from build123d import *

# Parameters (mm, degrees)
F0_W     = 169.7224378586
F0_H     = 29.1480664164
F1_DEPTH = 5
F2_R     = 5
F3_DEPTH = 5.001
F6_R     = 5
F7_DEPTH = 5


# Not quite as in the source:
# - a feature of the source that left no trace in its solid (it failed there, or was rolled back) is left out


with BuildPart() as f1:
    # F0 (on Top) → F1 (new body)
    with BuildSketch(Plane.XY):
        with Locations((-209.8612189293, 14.5740332082)):
            Rectangle(F0_W, F0_H)
        Polygon((125, -249.6209740639), (125, -125), (-125, -125), (-125, 0), (-294.7224378586, 0), (-294.7224378586, -249.6209740639), align=None)
        Polygon((124.7859969735, -298.5799014568), (125, -249.6209740639), (-294.7224378586, -249.6209740639), (-294.7224378586, -298.5799014568), align=None)
    extrude(amount=F1_DEPTH)

    # F2 (on face) → F3 (cut, through all)
    with BuildSketch(Plane.XY.offset(5)):
        with Locations((-228.7230412454, -24.2026941362)):
            Circle(F2_R)
        with Locations((-219.7715429866, -67.8267564705)):
            Circle(F2_R)
        with Locations((-202.5809461153, -108.9080358424)):
            Circle(F2_R)
        with Locations((-177.7957154285, -145.9064206102)):
            Circle(F2_R)
        with Locations((-146.3450338267, -177.4348643144)):
            Circle(F2_R)
        with Locations((-109.4079678244, -202.3113851876)):
            Circle(F2_R)
        with Locations((-68.3692650785, -219.6033779172)):
            Circle(F2_R)
        with Locations((-24.7674410595, -228.6625764382)):
            Circle(F2_R)
        with Locations((19.7628989378, -229.1493570263)):
            Circle(F2_R)
        with Locations((63.5523401318, -221.0454705796)):
            Circle(F2_R)
    extrude(amount=-F3_DEPTH, mode=Mode.SUBTRACT)


with BuildPart() as f7:
    # F6 (on face) → F7 (new body)
    with BuildSketch(Plane.XY.offset(5)):
        with BuildLine():
            ThreePointArc((-44.6295934942, -213.8640500528), (-51.5484234193, -191.3776944906), (-69.9114028179, -176.6703024168))
            ThreePointArc((-69.9114028179, -176.6703024168), (-121.8233411216, -199.1458593545), (-99.3477842144, -251.0577976715))
            ThreePointArc((-99.3477842144, -251.0577976715), (-62.1432379515, -246.945220141), (-44.6295934942, -213.8640500528))
        make_face()
        with Locations((-109.4079678244, -202.3113851876)):
            Circle(F6_R, mode=Mode.SUBTRACT)
        with Locations((-68.3692650785, -219.6033779172)):
            Circle(F6_R, mode=Mode.SUBTRACT)
        with BuildLine():
            ThreePointArc((-139.8690317235, -128.5949220021), (-132.0468964749, -141.1390217828), (-129.3151434854, -155.6675373561))
            ThreePointArc((-129.3151434854, -155.6675373561), (-154.7866291142, -192.9357848352), (-198.7612569937, -182.7401508106))
            ThreePointArc((-198.7612569937, -182.7401508106), (-152.9185251389, -222.5217397679), (-99.3477842144, -251.0577976715))
            ThreePointArc((-99.3477842144, -251.0577976715), (-121.8233411216, -199.1458593545), (-69.9114028179, -176.6703024168))
            ThreePointArc((-69.9114028179, -176.6703024168), (-107.6093315173, -156.5893731081), (-139.8690317235, -128.5949220021))
        make_face()
        with BuildLine():
            ThreePointArc((-198.7612569937, -182.7401508106), (-154.7866291142, -192.9357848352), (-129.3151434854, -155.6675373561))
            ThreePointArc((-129.3151434854, -155.6675373561), (-132.0468964749, -141.1390217828), (-139.8690317235, -128.5949220021))
            ThreePointArc((-139.8690317235, -128.5949220021), (-196.3877578897, -126.221424721), (-198.7612569937, -182.7401508106))
        make_face()
        with Locations((-146.3450338267, -177.4348643144)):
            Circle(F6_R, mode=Mode.SUBTRACT)
        with Locations((-177.7957154285, -145.9064206102)):
            Circle(F6_R, mode=Mode.SUBTRACT)
        with Locations((-109.4079678244, -202.3113851876)):
            Circle(F6_R)
        with Locations((-146.3450338267, -177.4348643144)):
            Circle(F6_R)
    extrude(amount=F7_DEPTH)


solid = f7.part
Design review of the part built by this model. Coordinates are the model's own, in mm. Round coordinates to 2 decimals unless told otherwise and drop trailing zeros. Write each loop counter-clockwise with the first axis right and the second up, starting at its lowest first coordinate (ties: lowest second). Pieces come first, ordered by that corner, then holes.
Item 1: For pin 1 Ø13 at (x, y) = (-68.37, -219.6) entering from +Z; pin 2 Ø3 at (y, z) = (-146, 6.5) entering from -X; pin 3 Ø3 at (x, z) = (-147.5, 6.5) entering from +Y, all flat-tipped, find the tip position at first contact; note any pin that passes through.
Item 2: Consider section D-D on y = -125. Give the boundary of the cut face in (x, z).
Item 3: Consider section A-A on x = -179. Give the boundary of the cut face in (y, z).
Item 4: Draft analysis for pull direction Y (two halves, no side actions). For faces 1 (the cylindrical face through (-63.75, -221.52, 7.46)), 2 (the cylindrical face through (-175.11, -141.69, 7.46)), 3 (the cylindrical face through (-195.73, -125.63, 7.46)), 4 (the flat face through (-128, -184, 10)), state which applies: released by +Y, released by -Y, zero draft, split by the parting line, or undercut.
Item 5: Consider section C-C on z = 7.8. Give the boundary of the cut face in (x, y).
Item 6: Wall thickness on L1, parallel to Y at x = -185, z = 8.2; L2, parallel to X at y = -195.5, z = 7.55 (3 decimals); L3, parallel to X at y = -150, z = 5.65: over which ranges is each line inside the solid? List them lowest first.
Item 7: Consider section B-B on y = -222. Give the boundary of the cut face in (x, z).
Check values:
1. pin 1: stops at z = 10
1. pin 2: stops at x = -208.47
1. pin 3: stops at y = -121.21
2. outline: (-195, 5) - (-143.63, 5) - (-143.63, 10) - (-195, 10) - close
3. outline: (-202.14, 5) - (-150.76, 5) - (-150.76, 10) - (-202.14, 10) - close; (-141.05, 5) - (-116.86, 5) - (-116.86, 10) - (-141.05, 10) - close
4. face 1: undercut
4. face 2: undercut
4. face 3: split by the parting line
4. face 4: zero draft
5. outline: (-198.76, -182.74) arc R270 ccw to (-99.35, -251.06) arc R40 ccw to (-69.91, -176.67) arc R190 cw to (-139.87, -128.59) arc R40 ccw to start; hole circle Ø10 at (-177.8, -145.91); hole circle Ø10 at (-68.37, -219.6)
6. L1: y = -196.66 to -118.87
6. L2: x = -186.225 to -49.094
6. L3: x = -208.91 to -180.67, -174.92 to -116.62
7. outline: (-153.67, 5) - (-72.76, 5) - (-72.76, 10) - (-153.67, 10) - close; (-63.98, 5) - (-45.47, 5) - (-45.47, 10) - (-63.98, 10) - close
